Could you check a few things on this model? Use its own coordinates, in mm. Face numbers are marked on the shaded views. A direction names the side the tool comes from. Coordinates: 2 decimals unless noted, no trailing zeros. Order: outer loops, then holes, each group sorted by start corner. A loop starts at its lowest first (then second) coordinate and runs counter-clockwise, first axis right, second up. Notation, with made-up numbers: M 56,89.25 L 113,89.25 A12 ccw 113,95.25 Z; hole C 47,38.25 d8. An arc over 180 degrees is marked long. Put each result on its own line as item: value. Start each with the question number.
```python
from build123d import *

# Parameters (mm, degrees)
F2_R     = 11.0758489904
F3_DEPTH = 114.3
F5_DEPTH = 469.9


with BuildPart() as f1:
    # F0 (on Front) → F1 (revolve)
    with BuildSketch(Plane.XZ):
        with BuildLine():
            Line((0, 89.3677696586), (0, 0))
            Line((0, 0), (20.591173321, 0))
            ThreePointArc((20.591173321, 0), (40.6415068424, 46.6066747904), (20.591173321, 93.2133495808))
            add(Edge.make_bspline(
                [(20.591173321, 93.2133495808), (18.7577284682, 89.4553018013), (15.1399751822, 82.0399221226), (11.807621021, 99.0461535157), (3.4854955303, 83.0706354136), (0.9970992228, 87.5663421121), (0, 89.3677696586)],
                knots=[0, 0, 0, 0, 0.261457833, 0.5159085822, 0.806024798, 1, 1, 1, 1], degree=3))
        make_face()
    revolve(axis=Axis((0, 0, 44.6838848293), (0, 0, -1)))

    # F2 (on Top) → F3 (join)
    with BuildSketch(Plane.XY):
        Circle(F2_R)
    extrude(amount=F3_DEPTH)

    # F4 (on Front) → F5 (cut, symmetric)
    with BuildSketch(Plane.XZ):
        Polygon((26.3139173462, 78.638642816), (15.4418259786, 83.8383438307), (5.502707124, 77.0226870214), (6.435679637, 65.0073291975), (17.3077710046, 59.8076281828), (27.2468898592, 66.6232849921), align=None)
        Polygon((7.7780308202, 29.657876119), (0, 41.9389754534), (-9.006138891, 29.657876119), align=None)
        with BuildLine():
            ThreePointArc((-18.4216499329, 18.1955154985), (-0.2779930332, 3.9861821268), (17.1935390681, 19.014256075))
            ThreePointArc((17.1935390681, 19.014256075), (-0.7270212138, 23.5188936817), (-18.4216499329, 18.1955154985))
        make_face()
        Polygon((-13.8043448256, 84.6826113726), (-24.6764361932, 77.794375274), (-24.1470944283, 64.9347499081), (-12.7456612958, 58.9633606408), (-1.8735699282, 65.8515967395), (-2.4029116931, 78.7112221054), align=None)
    extrude(amount=F5_DEPTH, both=True, mode=Mode.SUBTRACT)


solid = f1.part
```
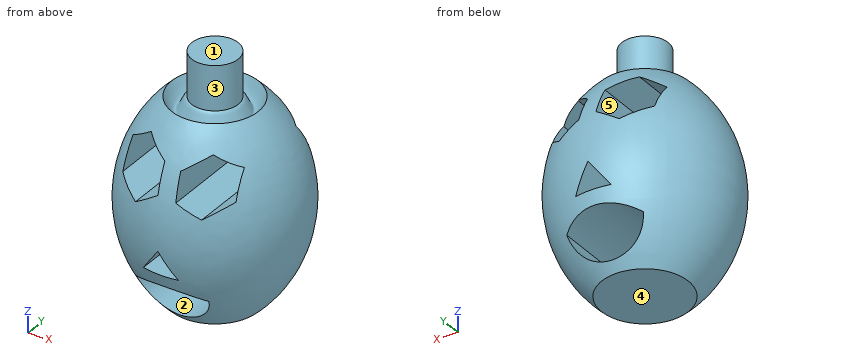
Item 1: For the marked faces 4 and 5, which set-ups out of +Z, -Z, +X, -X, +Y, -Y let a thin tool reach every point of the face, with its end or its side?
Item 2: For pin 1 Ø1.5 at (x, y) = (-11, -20) entering from -Z; pin 2 Ø1.5 at (y, z) = (-16.5, 93.5) entering from -X; pin 3 Ø3 at (x, z) = (7.5, 100.5) entering from -Y, each with a flat end and sliding along its axis, tell me the tip position at first contact or that it passes through.
Item 3: I need wall thicknesses on probe 1 along Z at (x, y) = (2, 9.5); probe 2 along X at (y, z) = (1, 79.5); probe 3 along Z at (x, y) = (2.5, 20). Which ranges of each line are inside material? Lowest first, please.
Item 4: If we section it at A-A on x = -4: State how many separate pieces and enclosed holes the cut face has, then the cut area to 3 significant figures.
Item 5: If we mould it in two halves opening along Z, with no side actions, what happens to the marked faces 1, 2 and 3? For each: released by +Z, released by -Z, zero draft, split by the parting line, or undercut.
Item 6: If we section it at C-C on z = 106.5: Write out the boundary of the cut face in (x, y), then the cut area to 3 significant figures.
Geometry check:
1. face 4: -Z, +X, -X, +Y, -Y
1. face 5: +Y, -Y
2. pin 1: stops at z = 1.45
2. pin 2: stops at x = -13.42
2. pin 3: stops at y = -9.31
3. probe 1: z = 0 to 4.18, 23.47 to 29.66, 38.78 to 114.3
3. probe 2: x = -31.56 to -21.98, -3.91 to 9.12, 24.51 to 31.56
3. probe 3: z = 0 to 4.26, 23.44 to 29.66, 37.99 to 92.32
4. separate pieces: 4
4. enclosed holes: 0
4. area: 3,980 mm²
5. face 1: released by +Z
5. face 2: undercut
5. face 3: zero draft
6. outline: C 0,0 d22.15
6. area: 385 mm²
